from build123d import *

# Parameters (mm, degrees)
CYLINDER_R     = 3
CYLINDER_DEPTH = 1
BOX_W          = 55
BOX_H          = 38
BOX_DEPTH      = 2
FILLET_R       = 6


with BuildPart() as cilindro:
    # Cylinder → Cylinder (new body)
    with BuildSketch(Plane(origin=(4, 16, 0), x_dir=(1, 0, 0), z_dir=(0, 0, 1))):
        Circle(CYLINDER_R)
    extrude(amount=CYLINDER_DEPTH)


with BuildPart() as cut002:
    # Box → Box (new body)
    with BuildSketch(Plane(origin=(-23.4593, -11.5423, 0), x_dir=(1, 0, 0), z_dir=(0, 0, 1))):
        with Locations((27.5, 19)):
            Rectangle(BOX_W, BOX_H)
    extrude(amount=BOX_DEPTH)

    # Fillet
    fillet_edges = [cut002.edges().sort_by_distance(p)[0] for p in [
        (-23.4593, -11.5423, 1),
        (-23.4593, 26.4577, 1),
        (31.5407, -11.5423, 1),
        (31.5407, 26.4577, 1),
    ]]
    fillet(fillet_edges, radius=FILLET_R)

    # Cut002: cut Cilindro
    add(cilindro.part, mode=Mode.SUBTRACT)


solid = cut002.part
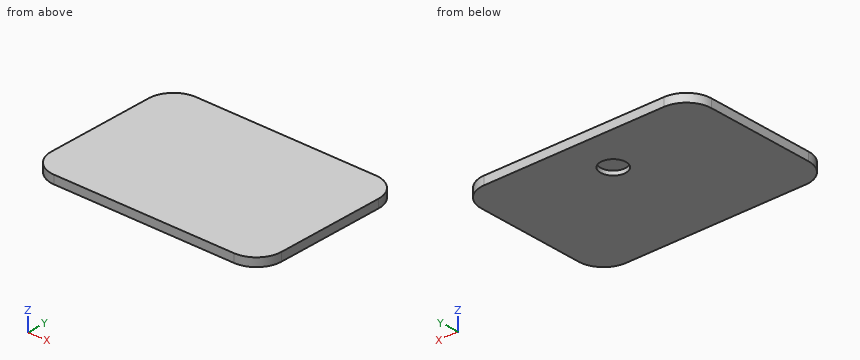
Source: CAD feature listing. Evaluate the final solid. Frame: model axes, mm. Round coordinates to 2 decimals unless told otherwise and drop trailing zeros. Order: outer loops, then holes, each group sorted by start corner. A loop starts at its lowest first (then second) coordinate and runs counter-clockwise, first axis right, second up. Notation, with made-up numbers: (-19.5, 24) - (19.5, 24) arc R19 cw to (19.5, 46) - close; hole circle Ø2 at (17.25, 87). An arc over 180 degrees is marked (long way). Use a Markdown table: item, result. Add a question column.
1. Section query B-B (y = 16). Return the cut outline in (x, z).
2. Line query: probe 1 along Y at (x, z) = (4, 0.6); probe 2 along X at (y, z) = (21, 1.1); probe 3 along X at (y, z) = (-10, 0.5). Output: solid intervals per line, ascending.
3. Section query A-A (z = 0.6). Return the cut outline in (x, y), then the cut area to 3 significant figures.
4. First-contact query: pin 1 (5 mm diameter, centred on x = 4.5, y = 17.5, fed in from -Z). Flat tip, straight axial feed; report the tip coordinate or a pass-through.
5. Section query C-C (x = 4). Return the cut outline in (y, z).
Derived:
| question | item | result |
|---|---|---|
| 1 | outline | (-23.46, 0) - (1, 0) - (1, 1) - (7, 1) - (7, 0) - (31.54, 0) - (31.54, 2) - (-23.46, 2) - close |
| 2 | probe 1 | -11.54 to 13, 19 to 26.46 |
| 2 | probe 2 | -23.43 to 31.52 |
| 2 | probe 3 | -21.48 to 29.56 |
| 3 | outline | (-23.46, -5.54) arc R6 ccw to (-17.46, -11.54) - (25.54, -11.54) arc R6 ccw to (31.54, -5.54) - (31.54, 20.46) arc R6 ccw to (25.54, 26.46) - (-17.46, 26.46) arc R6 ccw to (-23.46, 20.46) - close; hole circle Ø6 at (4, 16) |
| 3 | area | 2,030 mm2 |
| 4 | pin 1 | z = 0 |
| 5 | outline | (-11.54, 0) - (13, 0) - (13, 1) - (19, 1) - (19, 0) - (26.46, 0) - (26.46, 2) - (-11.54, 2) - close |
